Answer from the drawing. Dimensions are ordinates in mm from the lowest x, y and z of the part. Coordinates: 2 decimals unless noted, no trailing zeros. Order: outer loops, then holes, each group sorted by start corner. A loop starts at its lowest first (then second) coordinate and runs counter-clockwise, first axis right, second up. Notation, with made-up numbers: (-21, 5.5) - (-13, 5.5) arc R12 cw to (-13, 15.5) - close; hole circle Ø11 at (-23.5, 76.5). An arc over 180 degrees is marked (long way). Answer as a JSON object with one key per item and string values. Group by question number.
1) Find the intervals of material crossed by line 1 along Y through (x, z) = (51, 4.75) (1 decimal); line 2 along X through (y, z) = (43.5, 8.5) (1 decimal); line 3 along Y through (x, z) = (42, 8) (1 decimal), in increasing order.
2) Each of these flat-tipped pins is pushed along its axis until it touches: P1, Ø1, axis at x = 76, z = 5.5, coming from the +Y side; P2, Ø2, axis at x = 60.5, z = 2, coming from the +Y side; P3, Ø3, axis at x = 16, z = 5, coming from the -Y side. Where does it stop, or does it pass through?
3) Section A-A (z = 8) is taken. Give the vertices of the cut face in (x, y), plus the area to 3 significant figures.
4) Section C-C (x = 96.5) is taken. Give the vertices of the cut face in (y, z) (1 decimal).
5) Section B-B (x = 20) is taken. Give the vertices of the cut face in (y, z).
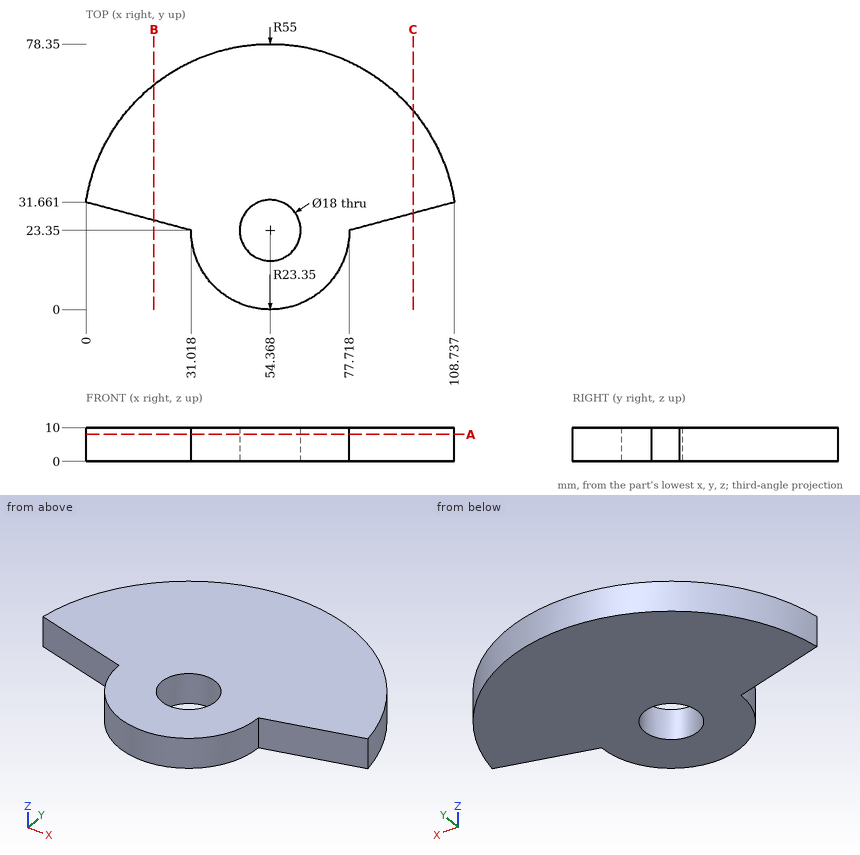
Report:
{
 "1": {"line 1": "y = 0.2 to 15, 31.7 to 78.2", "line 2": "x = 3.2 to 105.5", "line 3": "y = 3.5 to 76.9"},
 "2": {"P1": "stops at y = 74.13", "P2": "stops at y = 78.11", "P3": "stops at y = 26.97"},
 "3": {"outline": "(0, 31.66) - (31.02, 23.35) arc R23.35 ccw to (77.72, 23.35) - (108.74, 31.66) arc R55 ccw to start; hole circle Ø18 at (54.37, 23.35)", "area": "5,090 mm²"},
 "4": {"outline": "(28.4, 0) - (58.7, 0) - (58.7, 10) - (28.4, 10) - close"},
 "5": {"outline": "(26.3, 0) - (66.29, 0) - (66.29, 10) - (26.3, 10) - close"}
}
